Print and shaded views of the part. All mm, measured from the part's lowest x, y and z. A direction names the side the tool comes from. Coordinates: 2 decimals unless noted, no trailing zeros. Order: outer loops, then holes, each group sorted by start corner. A loop starts at its lowest first (then second) coordinate and runs counter-clockwise, first axis right, second up. Notation, with made-up numbers: (42.25, -13.75) -> (59.25, -13.75) arc R20 ccw to (59.25, 10.25) -> close; hole circle Ø2 at (49, 25.25). An arc over 180 degrees is marked (long way). Use one line per item in the form item = value. Start each with the question number.
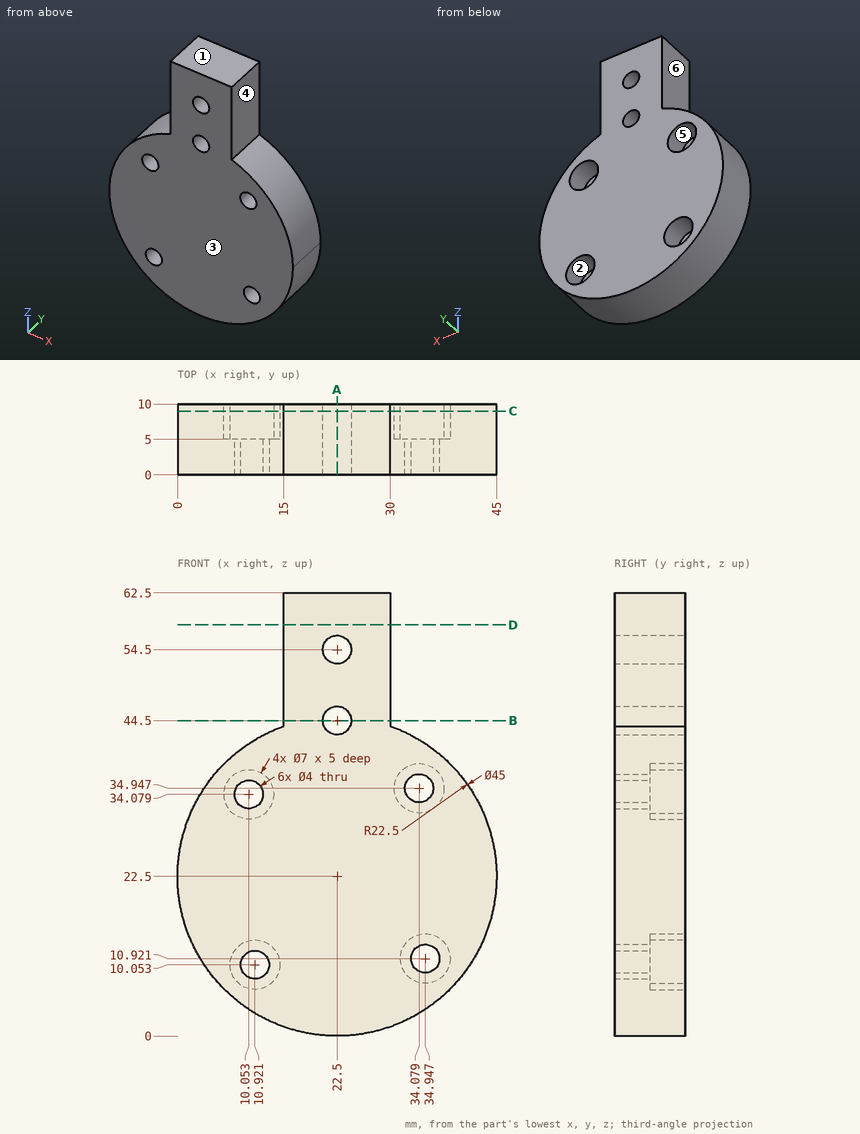
1) 3-axis set-ups, long thin cutter, end or side, ignore diameter. For the marked faces 4, 5 and 6: which of +Z, -Z, +X, -X, +Y, -Y reach the whole face in a straight line?
2) Probe L1, parallel to Z at x = 22.5, y = 6.5; L2, parallel to Z at x = 33, y = 8 (1 decimal); L3, parallel to X at y = 8.75, z = 32.5 (1 decimal). List the from-to ranges inside material, lowest first.
3) Cut at A-A on x = 22.5. Give the cut face in (y, z).
4) Cut at D-D on z = 58. Give the cut face in (x, y).
5) Cut at C-C on y = 9. Give the cut face in (x, z), then the cut area to 3 significant figures.
6) Cut at B-B on z = 44.5. Give the cut face in (x, y), then the cut area to 3 significant figures.
7) Two-plate mould, pull along Z, no slides. Class the marked faces 1, 2 and 3: released by +Z, released by -Z, zero draft, split by the parting line, or undercut.
8) Drop flat-ended pins along their axis: P1, Ø6, axis at y = 3.5, z = 16, coming from the -X side; P2, Ø5.5, axis at x = 10.5, z = 34.5, coming from the +Y side; P3, Ø5, axis at y = 2, z = 54.5, coming from the +X side. Give the stop position or say it passes through.
Values follow:
q1.face_4 = +Z, +X, +Y, -Y
q1.face_5 = +Y
q1.face_6 = +Z, -X, +Y, -Y
q2.L1 = 0 to 42.5, 46.5 to 52.5, 56.5 to 62.5
q2.L2 = 2.6 to 8, 13.8 to 31.6, 38.3 to 42.4
q2.L3 = 2.3 to 6.9, 13.2 to 31.6, 36.6 to 42.7
q3.outline = (0, 0) -> (10, 0) -> (10, 42.5) -> (0, 42.5) -> close; (0, 46.5) -> (10, 46.5) -> (10, 52.5) -> (0, 52.5) -> close; (0, 56.5) -> (10, 56.5) -> (10, 62.5) -> (0, 62.5) -> close
q4.outline = (15, 0) -> (30, 0) -> (30, 10) -> (15, 10) -> close
q5.outline = (15, 43.71) arc R22.5 ccw (long way) to (30, 43.71) -> (30, 62.5) -> (15, 62.5) -> close; hole circle Ø7 at (10.05, 34.08); hole circle Ø7 at (10.92, 10.05); hole circle Ø4 at (22.5, 44.5); hole circle Ø4 at (22.5, 54.5); hole circle Ø7 at (34.08, 34.95); hole circle Ø7 at (34.95, 10.92)
q5.area = 1,680 mm^2
q6.outline = (15, 0) -> (20.5, 0) -> (20.5, 10) -> (15, 10) -> close; (24.5, 0) -> (30, 0) -> (30, 10) -> (24.5, 10) -> close
q6.area = 110 mm^2
q7.face_1 = released by +Z
q7.face_2 = undercut
q7.face_3 = zero draft
q8.P1 = 0.27
q8.P2 = 5
q8.P3 = 30
